CAD build for the part. Positions are in the model's coordinates, mm. A direction names the side the tool comes from. Coordinates: 2 decimals unless noted, no trailing zeros. Loops run counter-clockwise (first coordinate to the right, second up) from the corner with the lowest first, then second, coordinate; pieces in that order, holes last. Notation, with made-up numbers: (51, -6) - (58, -6) arc R14 cw to (58, 20) - close; hole circle Ø8 at (85.5, -6.5). An arc over 180 degrees is marked (long way). Put each result on its own line as item: value.
```python
from build123d import *

# Parameters (mm, degrees)
CUT_EXTRUDE1_DEPTH = 10


with BuildPart() as part:
    # Sketch1 → Revolve1 (revolve)
    with BuildSketch(Plane.XY):
        Polygon((7.5, 0), (7.5, 8), (13.5, 8), (13.5, 6), (9.5, 6), (9.5, 0), align=None)
    revolve(axis=Axis((0, 0, 0), (0, 1, 0)))

    # Sketch2 → Cut-Extrude1 (cut)
    with BuildSketch(Plane(origin=(0, 0, 0), x_dir=(1, 0, 0), z_dir=(0, 1, 0))):
        Polygon((-9.091166867, -15.746362913), (0, 0), (8.625529774, -14.939855811), align=None)
    extrude(amount=CUT_EXTRUDE1_DEPTH, mode=Mode.SUBTRACT)


solid = part.part
```
Q1. Tool access for faces 4 (the cylindrical face through (0.49, 6.99, -13.49)), 5 (the cylindrical face through (0.348, 2.958, -9.494)), 6 (the flat face through (-4.6, 4.83, 7.97)): list every direction of +Z, -Z, +X, -X, +Y, -Y with a clear straight run to the whole face (end or side of a thin tool).
Determined:
face 4: +Y, -Y
face 5: -Y
face 6: +Z, +Y, -Y
Q2. Slice it at A-A, the plane z = 0. Give the cut face in (x, y), then the cut area to 3 significant figures.
Determined:
outline: (-13.5, 6) - (-9.5, 6) - (-9.5, 0) - (-7.5, 0) - (-7.5, 8) - (-13.5, 8) - close; (7.5, 0) - (9.5, 0) - (9.5, 6) - (13.5, 6) - (13.5, 8) - (7.5, 8) - close
area: 48.0 mm2
Q3. Pin check, flat tips, straight feed: pin 1 Ø4 at (y, z) = (3.5, -5) entering from -X; pin 2 Ø1.5 at (y, z) = (4.5, 7) entering from -X. Stop position of each tip, or through.
Determined:
pin 1: x = -9.01
pin 2: x = -7.15
Q4. Slice it at B-B, the plane x = 5.75. Give the cut face in (y, z).
Determined:
outline: (0, -7.56) - (6, -7.56) - (6, -12.21) - (8, -12.21) - (8, -4.82) - (0, -4.82) - close; (0, 4.82) - (8, 4.82) - (8, 9.96) - (6, 9.96) - (6, 7.56) - (0, 7.56) - close
Q5. Wall check: L1, parallel to Y at x = -10.75, z = 5.75; L2, parallel to X at y = 1.5, z = -1.5; L3, parallel to Z at x = 5.25, y = 5.75. Give the ranges that are in metal, low to high. Write a range as from..to.
Determined:
L1: 6..8
L2: -9.38..-7.35, 7.35..9.38
L3: -7.92..-5.36, 5.36..7.92
Q6. Slice it at D-D, the plane x = 0. Give the cut face in (y, z), then the cut area to 3 significant figures.
Determined:
outline: (0, -9.5) - (6, -9.5) - (6, -13.5) - (8, -13.5) - (8, -7.5) - (0, -7.5) - close
area: 24.0 mm2
Q7. Mould opens along Z. For faces 1 (the cylindrical face through (0.275, 4.056, -7.495)), 2 (the flat face through (-1, 0, -8)), 3 (the flat face through (4.56, 4.83, 7.9)) say: +Z half, -Z half, draft (parallel to the pull), parting line (faces both ways), or undercut.
Determined:
face 1: undercut
face 2: draft
face 3: +Z half
Q8. Slice it at C-C, the plane z = -9. Give the cut face in (x, y).
Determined:
outline: (-10.06, 6) - (-3.04, 6) - (-3.04, 0) - (3.04, 0) - (3.04, 6) - (10.06, 6) - (10.06, 8) - (-10.06, 8) - close
